Geometry: final body of the model. Coordinates: model frame, mm. Face numbers are marked on the shaded views. A direction names the side the tool comes from. Round coordinates to 2 decimals unless told otherwise and drop trailing zeros. Order: outer loops, then holes, each group sorted by start corner. A loop starts at its lowest first (then second) coordinate and runs counter-clockwise, first axis right, second up. Notation, with made-up numbers: (33.25, 7) - (88.25, 7) arc R24 ccw to (88.25, 30) - close; hole circle Ø3 at (-8.5, 13). An arc over 180 degrees is marked (long way). Put each result on its own line as item: value. Start each with the question number.
(1) Material intervals for L1, parallel to Y at x = 37.45, z = 51; L2, parallel to X at y = 0.7, z = 3; L3, parallel to X at y = 39, z = 88, sorted ascending. Write a range as [from, to].
(2) Section B-B (y = 26). Output: boundary loops of the cut face in (x, z).
(3) Access query for the marked faces 1 and 2. Directions: +Z, -Z, +X, -X, +Y, -Y. A direction counts if a zero-diameter tool reaches every point of the face in a straight line with its end or side. Return the directions, or none.
(4) Pin query (flat end, axial travel): P1, Ø3.5, axis at y = 9, z = 3, coming from the +X side; P2, Ø2.5, axis at y = 33, z = 87, coming from the +X side; P3, Ø3, axis at y = 39, z = 75, coming from the -X side; P4, Ø3.5, axis at x = 6, z = 3, coming from the +Y side. Return the tip coordinate at first contact, or that it passes through.
(5) Section A-A (z = 75). Count the separate pieces of the cut face and the enclosed holes in it, and give its area (3 significant figures).
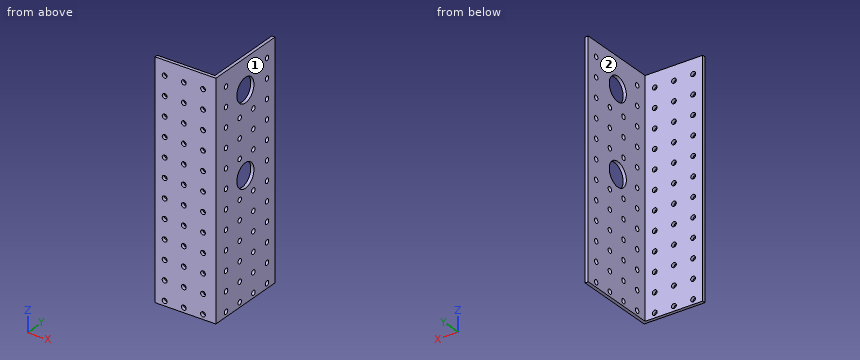
from build123d import *

# Parameters (mm, degrees)
SKETCH1_W           = 38
SKETCH1_H           = 150
SKETCH1_R           = 1.5
BOSS_EXTRUDE1_DEPTH = 2
SKETCH2_W           = 2
SKETCH2_H           = 150
BOSS_EXTRUDE2_DEPTH = 50
SKETCH3_R           = 1.5
SKETCH3_R_2         = 7.5
CUT_EXTRUDE1_DEPTH  = 50
CUT_EXTRUDE2_DEPTH  = 6


with BuildPart() as part:
    # Sketch1 → Boss-Extrude1 (new body)
    with BuildSketch(Plane(origin=(0, 0, 0), x_dir=(1, 0, 0), z_dir=(0, 1, 0))):
        with Locations((19, -75)):
            Rectangle(SKETCH1_W, SKETCH1_H)
        with Locations((6, -3)):
            Circle(SKETCH1_R, mode=Mode.SUBTRACT)
        with Locations((18, -3)):
            Circle(SKETCH1_R, mode=Mode.SUBTRACT)
        with Locations((30, -3)):
            Circle(SKETCH1_R, mode=Mode.SUBTRACT)
        with Locations((18, -15)):
            Circle(SKETCH1_R, mode=Mode.SUBTRACT)
        with Locations((30, -15)):
            Circle(SKETCH1_R, mode=Mode.SUBTRACT)
        with Locations((18, -27)):
            Circle(SKETCH1_R, mode=Mode.SUBTRACT)
        with Locations((30, -27)):
            Circle(SKETCH1_R, mode=Mode.SUBTRACT)
        with Locations((18, -39)):
            Circle(SKETCH1_R, mode=Mode.SUBTRACT)
        with Locations((30, -39)):
            Circle(SKETCH1_R, mode=Mode.SUBTRACT)
        with Locations((18, -51)):
            Circle(SKETCH1_R, mode=Mode.SUBTRACT)
        with Locations((30, -51)):
            Circle(SKETCH1_R, mode=Mode.SUBTRACT)
        with Locations((18, -63)):
            Circle(SKETCH1_R, mode=Mode.SUBTRACT)
        with Locations((30, -63)):
            Circle(SKETCH1_R, mode=Mode.SUBTRACT)
        with Locations((18, -75)):
            Circle(SKETCH1_R, mode=Mode.SUBTRACT)
        with Locations((30, -75)):
            Circle(SKETCH1_R, mode=Mode.SUBTRACT)
        with Locations((18, -87)):
            Circle(SKETCH1_R, mode=Mode.SUBTRACT)
        with Locations((30, -87)):
            Circle(SKETCH1_R, mode=Mode.SUBTRACT)
        with Locations((18, -99)):
            Circle(SKETCH1_R, mode=Mode.SUBTRACT)
        with Locations((30, -99)):
            Circle(SKETCH1_R, mode=Mode.SUBTRACT)
        with Locations((18, -111)):
            Circle(SKETCH1_R, mode=Mode.SUBTRACT)
        with Locations((30, -111)):
            Circle(SKETCH1_R, mode=Mode.SUBTRACT)
        with Locations((18, -123)):
            Circle(SKETCH1_R, mode=Mode.SUBTRACT)
        with Locations((30, -123)):
            Circle(SKETCH1_R, mode=Mode.SUBTRACT)
        with Locations((18, -135)):
            Circle(SKETCH1_R, mode=Mode.SUBTRACT)
        with Locations((30, -135)):
            Circle(SKETCH1_R, mode=Mode.SUBTRACT)
        with Locations((18, -147)):
            Circle(SKETCH1_R, mode=Mode.SUBTRACT)
        with Locations((30, -147)):
            Circle(SKETCH1_R, mode=Mode.SUBTRACT)
        with Locations((6, -15)):
            Circle(SKETCH1_R, mode=Mode.SUBTRACT)
        with Locations((6, -27)):
            Circle(SKETCH1_R, mode=Mode.SUBTRACT)
        with Locations((6, -39)):
            Circle(SKETCH1_R, mode=Mode.SUBTRACT)
        with Locations((6, -51)):
            Circle(SKETCH1_R, mode=Mode.SUBTRACT)
        with Locations((6, -63)):
            Circle(SKETCH1_R, mode=Mode.SUBTRACT)
        with Locations((6, -75)):
            Circle(SKETCH1_R, mode=Mode.SUBTRACT)
        with Locations((6, -87)):
            Circle(SKETCH1_R, mode=Mode.SUBTRACT)
        with Locations((6, -99)):
            Circle(SKETCH1_R, mode=Mode.SUBTRACT)
        with Locations((6, -111)):
            Circle(SKETCH1_R, mode=Mode.SUBTRACT)
        with Locations((6, -123)):
            Circle(SKETCH1_R, mode=Mode.SUBTRACT)
        with Locations((6, -135)):
            Circle(SKETCH1_R, mode=Mode.SUBTRACT)
        with Locations((6, -147)):
            Circle(SKETCH1_R, mode=Mode.SUBTRACT)
    extrude(amount=BOSS_EXTRUDE1_DEPTH)

    # Sketch2 → Boss-Extrude2 (add)
    with BuildSketch(Plane(origin=(0, 2, 0), x_dir=(1, 0, 0), z_dir=(0, 1, 0))):
        with Locations((37, -75)):
            Rectangle(SKETCH2_W, SKETCH2_H)
    extrude(amount=BOSS_EXTRUDE2_DEPTH)

    # Sketch3 → Cut-Extrude1 (cut)
    with BuildSketch(Plane(origin=(38, 0, 0), x_dir=(0, 0, -1), z_dir=(1, 0, 0))):
        with Locations((-147, 45)):
            Circle(SKETCH3_R)
        with Locations((-135, 45)):
            Circle(SKETCH3_R)
        with Locations((-123, 45)):
            Circle(SKETCH3_R)
        with Locations((-111, 45)):
            Circle(SKETCH3_R)
        with Locations((-99, 45)):
            Circle(SKETCH3_R)
        with Locations((-87, 45)):
            Circle(SKETCH3_R)
        with Locations((-75, 45)):
            Circle(SKETCH3_R)
        with Locations((-63, 45)):
            Circle(SKETCH3_R)
        with Locations((-51, 45)):
            Circle(SKETCH3_R)
        with Locations((-39, 45)):
            Circle(SKETCH3_R)
        with Locations((-27, 45)):
            Circle(SKETCH3_R)
        with Locations((-15, 45)):
            Circle(SKETCH3_R)
        with Locations((-3, 45)):
            Circle(SKETCH3_R)
        with Locations((-111, 33)):
            Circle(SKETCH3_R)
        with Locations((-99, 33)):
            Circle(SKETCH3_R)
        with Locations((-87, 33)):
            Circle(SKETCH3_R)
        with Locations((-63, 33)):
            Circle(SKETCH3_R)
        with Locations((-51, 33)):
            Circle(SKETCH3_R)
        with Locations((-39, 33)):
            Circle(SKETCH3_R)
        with Locations((-27, 33)):
            Circle(SKETCH3_R)
        with Locations((-3, 33)):
            Circle(SKETCH3_R)
        with Locations((-111, 21)):
            Circle(SKETCH3_R)
        with Locations((-99, 21)):
            Circle(SKETCH3_R)
        with Locations((-87, 21)):
            Circle(SKETCH3_R)
        with Locations((-63, 21)):
            Circle(SKETCH3_R)
        with Locations((-51, 21)):
            Circle(SKETCH3_R)
        with Locations((-39, 21)):
            Circle(SKETCH3_R)
        with Locations((-27, 21)):
            Circle(SKETCH3_R)
        with Locations((-3, 21)):
            Circle(SKETCH3_R)
        with Locations((-135, 9)):
            Circle(SKETCH3_R)
        with Locations((-123, 9)):
            Circle(SKETCH3_R)
        with Locations((-111, 9)):
            Circle(SKETCH3_R)
        with Locations((-99, 9)):
            Circle(SKETCH3_R)
        with Locations((-87, 9)):
            Circle(SKETCH3_R)
        with Locations((-75, 9)):
            Circle(SKETCH3_R)
        with Locations((-63, 9)):
            Circle(SKETCH3_R)
        with Locations((-51, 9)):
            Circle(SKETCH3_R)
        with Locations((-39, 9)):
            Circle(SKETCH3_R)
        with Locations((-27, 9)):
            Circle(SKETCH3_R)
        with Locations((-15, 9)):
            Circle(SKETCH3_R)
        with Locations((-3, 9)):
            Circle(SKETCH3_R)
        with Locations((-147, 33)):
            Circle(SKETCH3_R)
        with Locations((-147, 21)):
            Circle(SKETCH3_R)
        with Locations((-147, 9)):
            Circle(SKETCH3_R)
        with Locations((-75, 26)):
            Circle(SKETCH3_R_2)
        with Locations((-15, 21)):
            Circle(SKETCH3_R)
        with Locations((-15, 33)):
            Circle(SKETCH3_R)
        with Locations((-125, 26)):
            Circle(SKETCH3_R_2)
    extrude(amount=-CUT_EXTRUDE1_DEPTH, mode=Mode.SUBTRACT)

    # Sketch4 → Cut-Extrude2 (cut)
    with BuildSketch(Plane.XY.offset(150)):
        Polygon((0, 0), (38, 0), (38, 52), (36, 52), (36, 2), (0, 2), align=None)
    extrude(amount=-CUT_EXTRUDE2_DEPTH, mode=Mode.SUBTRACT)


solid = part.part
Checks:
1. L1: y = [0, 7.5], [10.5, 19.5], [22.5, 31.5], [34.5, 43.5], [46.5, 52]
1. L2: x = [0, 4.5], [7.5, 16.5], [19.5, 28.5], [31.5, 38]
1. L3: x = [36, 38]
2. outline: (36, 0) - (38, 0) - (38, 67.5) - (36, 67.5) - close; (36, 82.5) - (38, 82.5) - (38, 117.5) - (36, 117.5) - close; (36, 132.5) - (38, 132.5) - (38, 144) - (36, 144) - close
3. face 1: +Z, -Z, +X, +Y, -Y
3. face 2: +Z, -Z, -X, +Y
4. P1: stops at x = 38
4. P2: passes through
4. P3: stops at x = 36
4. P4: stops at y = 2
5. separate pieces: 7
5. enclosed holes: 0
5. area: 116 mm²
